Could you check a few things on this model? Use its own coordinates, in mm. A direction names the side the tool comes from. Round coordinates to 2 decimals unless told otherwise and drop trailing zeros. Order: outer loops, then holes, each group sorted by start corner. A loop starts at its lowest first (then second) coordinate and runs counter-clockwise, first axis right, second up. Notation, with made-up numbers: M -35.5,-29 L -4.5,-29 A20 ccw -4.5,-2 Z; hole C 16,19 d5. An arc over 180 degrees is marked long. Write each question's results on one line, items separated by ' | '. Start each with the question number.
1. Suppose I cut it at A-A on z = 13.25. Write out the boundary of the cut face in (x, y), and give its area (3 significant figures).
2. We'd pull the mould along Y, two halves only. Please class faces 4 (the flat face through (-3, 0, 20)), 5 (the flat face through (-22, 23, 5)), 6 (the cylindrical face through (-20.56, -4.27, 14.93)): released by +Y, released by -Y, zero draft, split by the parting line, or undercut.
3. Suppose I cut it at B-B on x = 24. Write out the boundary of the cut face in (y, z), and give its area (3 significant figures).
4. For faces 1 (the flat face through (12, 0, 15)), 2 (the flat face through (13, 2, 20)), 3 (the flat face through (20, 4, 15)), which set-ups out of +Z, -Z, +X, -X, +Y, -Y let a thin tool reach every point of the face, with its end or its side?
5. Suppose I cut it at C-C on y = 23. Write out the boundary of the cut face in (x, z).
6. I'm going to push flat-ended pins straight in: pin 1 (2 mm diameter, centred on y = -8, z = 13.5, fed in from +X); pin 2 (6 mm diameter, centred on y = -19.5, z = 15.5, fed in from +X); pin 3 (6 mm diameter, centred on x = -20.5, z = 17.5, fed in from +Y). Where does each tip first touch, or does it pass through?
7. Please list where these lines run through material, in increasing order: L1, parallel to X at y = 0, z = 13.25; L2, parallel to X at y = 8, z = 11.5; L3, parallel to Y at x = 0, z = 12.5.
8. Suppose I cut it at D-D on z = 7. Write out the boundary of the cut face in (x, y).
from build123d import *

# Parameters (mm, degrees)
F1_DEPTH = 10
F3_DEPTH = 10
F5_DEPTH = 10


with BuildPart() as f1:
    # F0 (on Top) → F1 (new body)
    with BuildSketch(Plane.XY):
        Polygon((45, 0), (0, 45), (-45, 0), (0, -45), align=None)
    extrude(amount=F1_DEPTH)

    # F2 (on face) → F3 (join)
    with BuildSketch(Plane.XY.offset(10)):
        with BuildLine():
            Line((18.186533, 10.5), (25.114737, 14.5))
            ThreePointArc((25.114737, 14.5), (-27.425954, -9.42428), (28.722813, 4))
            Line((28.722813, 4), (12, 4))
            Line((12, 4), (12, -4))
            Line((12, -4), (20.615528, -4))
            ThreePointArc((20.615528, -4), (-20.71141, -3.469511), (18.186533, 10.5))
        make_face()
    extrude(amount=F3_DEPTH)

    # F4 (on face) → F5 (join)
    with BuildSketch(Plane.XY.offset(10)):
        with BuildLine():
            Line((3.5, 0), (14.5, 10.665365))
            ThreePointArc((14.5, 10.665365), (11.754954, 13.631619), (8.417301, 15.910658))
            Line((8.417301, 15.910658), (-5.5, 2.416741))
            Line((-5.5, 2.416741), (-5.5, -2.416741))
            Line((-5.5, -2.416741), (8.417301, -15.910658))
            ThreePointArc((8.417301, -15.910658), (11.754954, -13.631619), (14.5, -10.665365))
            Line((14.5, -10.665365), (3.5, 0))
        make_face()
        with BuildLine():
            Line((-5.5, -2.416741), (-5.5, 2.416741))
            Line((-5.5, 2.416741), (-5.5, 17.139137))
            ThreePointArc((-5.5, 17.139137), (-9.853768, 15.063308), (-13.5, 11.905881))
            Line((-13.5, 11.905881), (-13.5, -11.905881))
            ThreePointArc((-13.5, -11.905881), (-9.853768, -15.063308), (-5.5, -17.139137))
            Line((-5.5, -17.139137), (-5.5, -2.416741))
        make_face()
    extrude(amount=F5_DEPTH)


solid = f1.part
Filled sheet:
1) outline: M -13.5,-11.91 A18 ccw -5.5,-17.14 L -5.5,-2.42 L 8.42,-15.91 A18 ccw 14.5,-10.67 L 3.5,0 L 14.5,10.67 A18 ccw 8.42,15.91 L -5.5,2.42 L -5.5,17.14 A18 ccw -13.5,11.91 Z; M 12,-4 L 20.62,-4 A21 cw long 18.19,10.5 L 25.11,14.5 A29 ccw long 28.72,4 L 12,4 Z | area: 1,800 mm^2
2) face 4: zero draft | face 5: released by +Y | face 6: undercut
3) outline: M -21,0 L 21,0 L 21,10 L 16.28,10 L 16.28,20 L 13.86,20 L 13.86,10 L 4,10 L 4,20 L -16.28,20 L -16.28,10 L -21,10 Z | area: 647 mm^2
4) face 1: +Z | face 2: +Z, +X, -X, +Y, -Y | face 3: +Z, +X
5) outline: M -22,0 L 22,0 L 22,10 L 17.66,10 L 17.66,20 L -17.66,20 L -17.66,10 L -22,10 Z
6) pin 1: stops at x = 28.14 | pin 2: stops at x = 23.85 | pin 3: stops at y = 23.12
7) L1: x = -29 to -21, -13.5 to 3.5, 12 to 29 | L2: x = -27.87 to -19.42, -13.5 to -5.5, 0.26 to 11.75 | L3: y = -29 to -21, -7.75 to 7.75, 21 to 29
8) outline: M -45,0 L 0,-45 L 45,0 L 0,45 Z
